```python
from build123d import *

# Parameters (mm, degrees)
F1_DEPTH = 1
F2_R     = 0.5


with BuildPart() as f1:
    # F0 (on Front) → F1 (new body)
    with BuildSketch(Plane.XZ):
        with BuildLine():
            ThreePointArc((0.85, 2.981191), (0, -3.1), (-0.85, 2.981191))
            Line((-0.85, 2.981191), (-0.85, 9.764079))
            ThreePointArc((-0.85, 9.764079), (-1.5, 11), (-0.85, 12.235921))
            Line((-0.85, 12.235921), (-0.85, 13.5))
            Line((-0.85, 13.5), (-3, 13.5))
            Line((-3, 13.5), (-5, 9))
            Line((-5, 9), (-5, 0))
            ThreePointArc((-5, 0), (0, -5), (5, 0))
            Line((5, 0), (5, 9))
            Line((5, 9), (3, 13.5))
            Line((3, 13.5), (0.85, 13.5))
            Line((0.85, 13.5), (0.85, 12.235921))
            ThreePointArc((0.85, 12.235921), (1.5, 11), (0.85, 9.764079))
            Line((0.85, 9.764079), (0.85, 2.981191))
        make_face()
    extrude(amount=F1_DEPTH)

    # F2
    f2_edges = [f1.edges().sort_by_distance(p)[0] for p in [
        (3, -0.5, 13.5),
        (0.85, -0.5, 13.5),
        (-0.85, -0.5, 13.5),
        (-3, -0.5, 13.5),
        (-5, -0.5, 9),
        (5, -0.5, 9),
    ]]
    fillet(f2_edges, radius=F2_R)


solid = f1.part
```
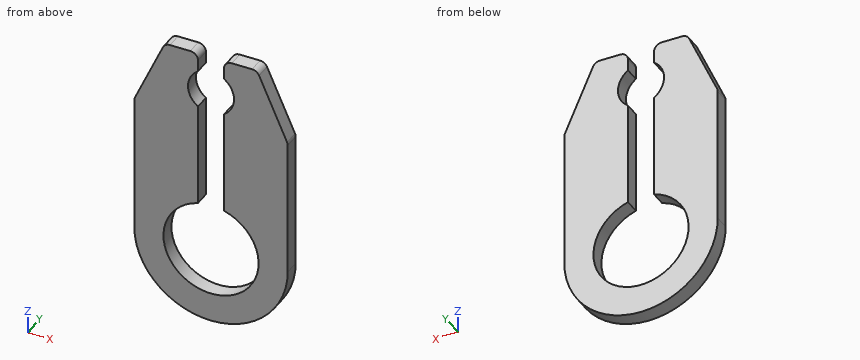
CAD build for the part. Positions are in the model's coordinates, mm. Coordinates: 2 decimals unless noted, no trailing zeros. Loops run counter-clockwise (first coordinate to the right, second up) from the corner with the lowest first, then second, coordinate; pieces in that order, holes last. Notation, with made-up numbers: (21.5, -6.75) - (32.5, -6.75) arc R19 ccw to (32.5, 17.25) - close; hole circle Ø11 at (67, 16). An arc over 180 degrees is marked (long way). Return JSON: item names as keys, results as strings.
1. Band-saw the part on A-A (z = 6.5). Give the cut face in (x, y), and give its area (3 significant figures).
Result:
{"outline": "(-5, -1) - (-0.85, -1) - (-0.85, 0) - (-5, 0) - close; (0.85, -1) - (5, -1) - (5, 0) - (0.85, 0) - close", "area": "8.30 mm2"}
2. Probe L1, parallel to X at y = -0.85, z = 3.75; L2, parallel to X at y = -0.8, z = 0; L3, parallel to Z at x = 1, y = -0.7. List the from-to ranges inside material, lowest first. Write a range as from..to.
Result:
{"L1": "x = -5..-0.85, 0.85..5", "L2": "x = -5..-3.1, 3.1..5", "L3": "z = -4.9..-2.93, 2.93..9.88, 12.12..13.36"}
3. Band-saw the part on C-C (z = 10.75). Give the cut face in (x, y), and give its area (3 significant figures).
Result:
{"outline": "(-4.22, -1) - (-1.48, -1) - (-1.48, 0) - (-4.22, 0) - close; (1.48, -1) - (4.22, -1) - (4.22, 0) - (1.48, 0) - close", "area": "5.49 mm2"}
4. Band-saw the part on B-B (y = -0.5). Give the cut face in (x, z), and give its area (3 significant figures).
Result:
{"outline": "(-5, 0) arc R5 ccw to (5, 0) - (5, 8.89) arc R0.5 ccw to (4.96, 9.1) - (3.13, 13.2) arc R0.5 ccw to (2.68, 13.5) - (1.35, 13.5) arc R0.5 ccw to (0.85, 13) - (0.85, 12.24) arc R1.5 cw to (0.85, 9.76) - (0.85, 2.98) arc R3.1 cw (long way) to (-0.85, 2.98) - (-0.85, 9.76) arc R1.5 cw to (-0.85, 12.24) - (-0.85, 13) arc R0.5 ccw to (-1.35, 13.5) - (-2.68, 13.5) arc R0.5 ccw to (-3.13, 13.2) - (-4.96, 9.1) arc R0.5 ccw to (-5, 8.89) - close", "area": "115 mm2"}
5. Band-saw the part on D-D (x = 0). Give the cut face in (y, z), and give its area (3 significant figures).
Result:
{"outline": "(-1, -5) - (0, -5) - (0, -3.1) - (-1, -3.1) - close", "area": "1.90 mm2"}
6. Drop flat-ended pins along their axis: pin 1 (0.6 mm diameter, centred on y = -0.5, z = 12.5, fed in from -X); pin 2 (0.6 mm diameter, centred on y = -0.5, z = 13, fed in from +X). Give the stop position or say it passes through.
Result:
{"pin 1": "stops at x = -3.58", "pin 2": "stops at x = 3.36"}
